Could you check a few things on this model? Use its own coordinates, in mm. Face numbers are marked on the shaded views. Round coordinates to 2 decimals unless told otherwise and drop trailing zeros. Loops run counter-clockwise (first coordinate to the right, second up) from the corner with the lowest first, then second, coordinate; pieces in that order, holes last. Notation, with made-up numbers: (51, 54) - (68, 54) arc R17 cw to (68, 82) - close; hole circle Ø9 at (83.5, -7.5). An arc over 180 degrees is marked (long way). Put each result on its own line as item: value. Start each with the question number.
from build123d import *

# Parameters (mm, degrees)
SKETCH1_R           = 46.5
SKETCH1_R_2         = 6.5
SKETCH1_R_3         = 10
SKETCH1_R_4         = 3.5
BOSS_EXTRUDE1_DEPTH = 2
SKETCH3_R           = 5
SKETCH3_R_2         = 3.5
BOSS_EXTRUDE2_DEPTH = 100
SKETCH4_R           = 30
SKETCH4_R_2         = 29
BOSS_EXTRUDE5_DEPTH = 2
FILLET2_R           = 2
SKETCH5_R           = 1
SKETCH5_R_2         = 3.5
CUT_EXTRUDE1_DEPTH  = 1
SKETCH6_R           = 2
CUT_EXTRUDE2_DEPTH  = 2
CHAMFER2_SIZE       = 0.8
SKETCH7_R           = 61.085714235
CUT_EXTRUDE3_DEPTH  = 122.361031637


with BuildPart() as part:
    # Sketch1 → Boss-Extrude1 (new body)
    with BuildSketch(Plane(origin=(0, 0, 0), x_dir=(1, 0, 0), z_dir=(0, 1, 0))):
        with Locations(Location((0, 0, 0), (0, 0, 270))):
            Circle(SKETCH1_R)
        with Locations(Location((0, 15, 0), (0, 0, 270))):
            Circle(SKETCH1_R_2, mode=Mode.SUBTRACT)
        with Locations(Location((-12.990381057, -7.5, 0), (0, 0, 270))):
            Circle(SKETCH1_R_3, mode=Mode.SUBTRACT)
        with Locations(Location((12.990381057, -7.5, 0), (0, 0, 270))):
            Circle(SKETCH1_R_4, mode=Mode.SUBTRACT)
        with Locations(Location((0, 0, 0), (0, 0, 270))):
            Circle(SKETCH1_R_4, mode=Mode.SUBTRACT)
    extrude(amount=BOSS_EXTRUDE1_DEPTH)

    # Sketch3 → Boss-Extrude2 (add)
    with BuildSketch(Plane(origin=(0, 2, 0), x_dir=(1, 0, 0), z_dir=(0, 1, 0))):
        with Locations(Location((0, 0, 0), (0, 0, 210))):
            Circle(SKETCH3_R)
        with Locations(Location((0, 0, 0), (0, 0, 270))):
            Circle(SKETCH3_R_2, mode=Mode.SUBTRACT)
    extrude(amount=BOSS_EXTRUDE2_DEPTH)

    # Sketch6 → Cut-Extrude2 (cut)
    with BuildSketch(Plane.XZ):
        with Locations(Location((0, 35, 0), (0, 0, 270))):
            Circle(SKETCH6_R)
        with Locations(Location((27.364101886, 21.822143065, 0), (0, 0, 270))):
            Circle(SKETCH6_R)
        with Locations(Location((34.122476926, -7.788232688, 0), (0, 0, 270))):
            Circle(SKETCH6_R)
        with Locations(Location((15.185930869, -31.533910377, 0), (0, 0, 270))):
            Circle(SKETCH6_R)
        with Locations(Location((-15.185930869, -31.533910377, 0), (0, 0, 270))):
            Circle(SKETCH6_R)
        with Locations(Location((-34.122476926, -7.788232688, 0), (0, 0, 270))):
            Circle(SKETCH6_R)
        with Locations(Location((-27.364101886, 21.822143065, 0), (0, 0, 270))):
            Circle(SKETCH6_R)
    extrude(amount=-CUT_EXTRUDE2_DEPTH, mode=Mode.SUBTRACT)

    # Chamfer2
    chamfer2_edges = [part.edges().sort_by_distance(p)[0] for p in [
        (12.990381057, 0, 4),
        (34.122476926, 0, -5.788232688),
        (27.364101886, 0, 23.822143065),
        (0, 0, 37),
        (-27.364101886, 0, 23.822143065),
        (-34.122476926, 0, -5.788232688),
        (-15.185930869, 0, -29.533910377),
        (15.185930869, 0, -29.533910377),
    ]]
    chamfer(chamfer2_edges, length=CHAMFER2_SIZE)

    # Sketch7 → Cut-Extrude3 (cut, through all)
    with BuildSketch(Plane.XZ.offset(-102)):
        Circle(SKETCH7_R)
    extrude(amount=CUT_EXTRUDE3_DEPTH, mode=Mode.SUBTRACT)


with BuildPart() as body_2:
    # Sketch4 → Boss-Extrude5 (new body)
    # profile 1 of 11: a face of its own
    with BuildSketch(Plane(origin=(0, 102, 0), x_dir=(1, 0, 0), z_dir=(0, 1, 0))):
        with Locations(Location((0, 0, 0), (0, 0, 270))):
            Circle(SKETCH4_R)
        Circle(SKETCH4_R_2, mode=Mode.SUBTRACT)
    # profile 2 of 11: a face of its own
    with BuildSketch(Plane(origin=(0, 102, 0), x_dir=(1, 0, 0), z_dir=(0, 1, 0))):
        with BuildLine():
            ThreePointArc((0.372035902, 9.373321886), (-3.288218135, 5.713067848), (-8.288218135, 4.373321886))
            Line((-8.288218135, 4.373321886), (-28.668345883, 4.373321886))
            ThreePointArc((-28.668345883, 4.373321886), (-29, 0), (-28.668345883, -4.373321886))
            Line((-28.668345883, -4.373321886), (-8.209333805, -4.373321886))
            ThreePointArc((-8.209333805, -4.373321886), (-3.209333805, -5.713067848), (0.450920232, -9.373321886))
            Line((0.450920232, -9.373321886), (10.619428606, -26.985695027))
            ThreePointArc((10.619428606, -26.985695027), (14.567551204, -25.075614687), (18.182472179, -22.591983212))
            Line((18.182472179, -22.591983212), (7.986293771, -4.931684166))
            ThreePointArc((7.986293771, -4.931684166), (6.646547809, 0.068315834), (7.986293771, 5.068315834))
            Line((7.986293771, 5.068315834), (18.128572143, 22.635257278))
            ThreePointArc((18.128572143, 22.635257278), (14.507755353, 25.110257558), (10.555107028, 27.010918452))
            Line((10.555107028, 27.010918452), (0.372035902, 9.373321886))
        make_face()
        with BuildLine():
            ThreePointArc((-4.421197961, -2.542244793), (-5.099992146, 0.008950407), (-4.412247554, 2.557747353))
            ThreePointArc((-4.412247554, 2.557747353), (-2.542244793, 4.421197961), (0.008950407, 5.099992146))
            ThreePointArc((0.008950407, 5.099992146), (2.557747353, 4.412247554), (4.421197961, 2.542244793))
            ThreePointArc((4.421197961, 2.542244793), (4.927378086, 1.315653905), (5.1, 0))
            ThreePointArc((5.1, 0), (4.925061549, -1.324299338), (4.412247554, -2.557747353))
            ThreePointArc((4.412247554, -2.557747353), (2.542244793, -4.421197961), (-0.008950407, -5.099992146))
            ThreePointArc((-0.008950407, -5.099992146), (-2.557747353, -4.412247554), (-4.421197961, -2.542244793))
        make_face(mode=Mode.SUBTRACT)
    # profile 3 of 11: a face of its own
    with BuildSketch(Plane(origin=(0, 102, 0), x_dir=(1, 0, 0), z_dir=(0, 1, 0))):
        with BuildLine():
            Line((-0.008950407, -5.099992146), (-0.008774909, -4.9999923))
            ThreePointArc((-0.008774909, -4.9999923), (-2.507595444, -4.325732896), (-4.334507805, -2.492396856))
            Line((-4.334507805, -2.492396856), (-4.421197961, -2.542244793))
            ThreePointArc((-4.421197961, -2.542244793), (-2.557747353, -4.412247554), (-0.008950407, -5.099992146))
        make_face()
    # profile 4 of 11: a face of its own
    with BuildSketch(Plane(origin=(0, 102, 0), x_dir=(1, 0, 0), z_dir=(0, 1, 0))):
        with BuildLine():
            Line((-4.412247554, 2.557747353), (-4.325732896, 2.507595444))
            ThreePointArc((-4.325732896, 2.507595444), (-2.492396856, 4.334507805), (0.008774909, 4.9999923))
            Line((0.008774909, 4.9999923), (0.008950407, 5.099992146))
            ThreePointArc((0.008950407, 5.099992146), (-2.542244793, 4.421197961), (-4.412247554, 2.557747353))
        make_face()
    # profile 5 of 11: a face of its own
    with BuildSketch(Plane(origin=(0, 102, 0), x_dir=(1, 0, 0), z_dir=(0, 1, 0))):
        with BuildLine():
            Line((4.421197961, 2.542244793), (4.334507805, 2.492396856))
            ThreePointArc((4.334507805, 2.492396856), (4.830762829, 1.28985677), (5, 0))
            ThreePointArc((5, 0), (4.828491715, -1.298332685), (4.325732896, -2.507595444))
            Line((4.325732896, -2.507595444), (4.412247554, -2.557747353))
            ThreePointArc((4.412247554, -2.557747353), (4.925061549, -1.324299338), (5.1, 0))
            ThreePointArc((5.1, 0), (4.927378086, 1.315653905), (4.421197961, 2.542244793))
        make_face()
    # profile 6 of 11: a face of its own
    with BuildSketch(Plane(origin=(0, 102, 0), x_dir=(1, 0, 0), z_dir=(0, 1, 0))):
        with BuildLine():
            ThreePointArc((-4.334507805, -2.492396856), (-4.9999923, 0.008774909), (-4.325732896, 2.507595444))
            Line((-4.325732896, 2.507595444), (-4.412247554, 2.557747353))
            ThreePointArc((-4.412247554, 2.557747353), (-5.099992146, 0.008950407), (-4.421197961, -2.542244793))
            Line((-4.421197961, -2.542244793), (-4.334507805, -2.492396856))
        make_face()
    # profile 7 of 11: a face of its own
    with BuildSketch(Plane(origin=(0, 102, 0), x_dir=(1, 0, 0), z_dir=(0, 1, 0))):
        with BuildLine():
            Line((4.412247554, -2.557747353), (4.325732896, -2.507595444))
            ThreePointArc((4.325732896, -2.507595444), (2.492396856, -4.334507805), (-0.008774909, -4.9999923))
            Line((-0.008774909, -4.9999923), (-0.008950407, -5.099992146))
            ThreePointArc((-0.008950407, -5.099992146), (2.542244793, -4.421197961), (4.412247554, -2.557747353))
        make_face()
    # profile 8 of 11: a face of its own
    with BuildSketch(Plane(origin=(0, 102, 0), x_dir=(1, 0, 0), z_dir=(0, 1, 0))):
        with BuildLine():
            Line((0.008950407, 5.099992146), (0.008774909, 4.9999923))
            ThreePointArc((0.008774909, 4.9999923), (2.507595444, 4.325732896), (4.334507805, 2.492396856))
            Line((4.334507805, 2.492396856), (4.421197961, 2.542244793))
            ThreePointArc((4.421197961, 2.542244793), (2.557747353, 4.412247554), (0.008950407, 5.099992146))
        make_face()
    # profile 9 of 11: a face of its own
    with BuildSketch(Plane(origin=(0, 102, 0), x_dir=(1, 0, 0), z_dir=(0, 1, 0))):
        with BuildLine():
            Line((-4.325732896, 2.507595444), (-3.028013027, 1.755316811))
            ThreePointArc((-3.028013027, 1.755316811), (-1.744677799, 3.034155464), (0.006142436, 3.49999461))
            Line((0.006142436, 3.49999461), (0.008774909, 4.9999923))
            ThreePointArc((0.008774909, 4.9999923), (-2.492396856, 4.334507805), (-4.325732896, 2.507595444))
        make_face()
    # profile 10 of 11: a face of its own
    with BuildSketch(Plane(origin=(0, 102, 0), x_dir=(1, 0, 0), z_dir=(0, 1, 0))):
        with BuildLine():
            Line((-0.008774909, -4.9999923), (-0.006142436, -3.49999461))
            ThreePointArc((-0.006142436, -3.49999461), (-1.755316811, -3.028013027), (-3.034155464, -1.744677799))
            Line((-3.034155464, -1.744677799), (-4.334507805, -2.492396856))
            ThreePointArc((-4.334507805, -2.492396856), (-2.507595444, -4.325732896), (-0.008774909, -4.9999923))
        make_face()
    # profile 11 of 11: a face of its own
    with BuildSketch(Plane(origin=(0, 102, 0), x_dir=(1, 0, 0), z_dir=(0, 1, 0))):
        with BuildLine():
            Line((4.334507805, 2.492396856), (3.034155464, 1.744677799))
            ThreePointArc((3.034155464, 1.744677799), (3.38153398, 0.902899739), (3.5, 0))
            ThreePointArc((3.5, 0), (3.3799442, -0.908832879), (3.028013027, -1.755316811))
            Line((3.028013027, -1.755316811), (4.325732896, -2.507595444))
            ThreePointArc((4.325732896, -2.507595444), (4.828491715, -1.298332685), (5, 0))
            ThreePointArc((5, 0), (4.830762829, 1.28985677), (4.334507805, 2.492396856))
        make_face()
    extrude(amount=BOSS_EXTRUDE5_DEPTH)

    # Fillet2
    fillet2_edges = [body_2.edges().sort_by_distance(p)[0] for p in [
        (10.555107028, 103, -27.010918452),
        (-28.668345883, 103, -4.373321886),
        (18.128572143, 103, -22.635257278),
        (18.182472179, 103, 22.591983212),
        (10.619428606, 103, 26.985695027),
        (-28.668345883, 103, 4.373321886),
    ]]
    fillet(fillet2_edges, radius=FILLET2_R)

    # Sketch5 → Cut-Extrude1 (cut)
    with BuildSketch(Plane.XZ.offset(-102)):
        with Locations(Location((-15, 0, 0), (0, 0, 270))):
            Circle(SKETCH5_R)
        with Locations(Location((7.5, 12.990381057, 0), (0, 0, 270))):
            Circle(SKETCH5_R_2)
        Polygon((8.383974596, -16.52146997), (4.883974596, -10.459292144), (6.616025404, -9.459292144), (10.116025404, -15.52146997), align=None)
    extrude(amount=-CUT_EXTRUDE1_DEPTH, mode=Mode.SUBTRACT)


solid = body_2.part
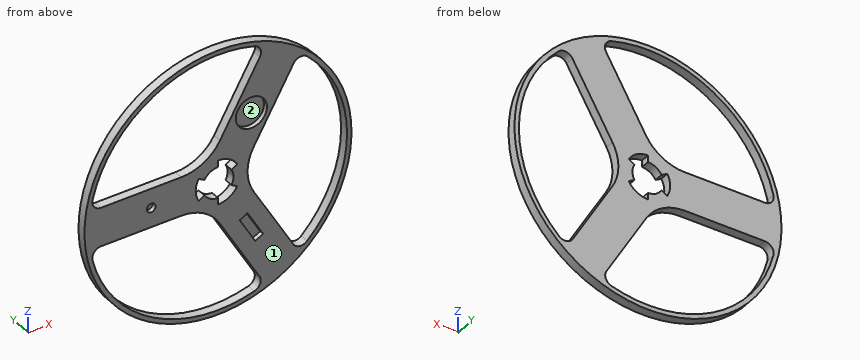
Item 1: Suppose I cut it at B-B, the plane z = 6. List the corners of the cut face in (x, y) for me.
Item 2: Suppose I cut it at C-C, the plane x = -15. List the corners of the cut face in (y, z) for me.
Item 3: Suppose I cut it at A-A, the plane x = -6. List the corners of the cut face in (y, z) for me, then the cut area to 3 significant figures.
Item 4: Thinking about a two-plate mould opening in X: for the marked faces 1 and 2, which applies, released by +X, released by -X, zero draft, split by the parting line, or undercut?
Item 5: Will these pins go through, and if not, where does the flat tip stop? P1, Ø5.5, axis at x = 7, z = 12.5, coming from the -Y side; P2, Ø2.5, axis at x = 7, z = -12.5, coming from the -Y side; P3, Ø1, axis at y = 103, z = 6.5, coming from the -X side.
Item 6: I need wall thicknesses on line 1 (X direction, y = 102.5, z = 17); line 2 (Z direction, x = 8.5, y = 103.5); line 3 (Z direction, x = -18, y = 102.1). Which ranges of each line are inside material? Lowest first, please. Write a range as from..to.
Numbers:
1. outline: (-29.39, 102) - (-28.2, 102) - (-28.2, 104) - (-29.39, 104) - close; (-2.74, 102) - (8.6, 102) - (8.6, 104) - (-2.74, 104) - close; (28.37, 102) - (29.39, 102) - (29.39, 104) - (28.37, 104) - close
2. outline: (102, -25.98) - (104, -25.98) - (104, -24.82) - (102, -24.82) - close; (102, -4.37) - (104, -4.37) - (104, 4.37) - (102, 4.37) - (102, 1) - (103, 1) - (103, -1) - (102, -1) - close; (102, 24.82) - (104, 24.82) - (104, 25.98) - (102, 25.98) - close
3. outline: (102, -29.39) - (104, -29.39) - (104, -28.37) - (102, -28.37) - close; (102, -4.64) - (104, -4.64) - (104, 4.62) - (102, 4.62) - close; (102, 28.37) - (104, 28.37) - (104, 29.39) - (102, 29.39) - close
3. area: 22.6 mm^2
4. face 1: zero draft
4. face 2: undercut
5. P1: y = 103
5. P2: y = 102
5. P3: x = -29.39
6. line 1: -24.72..-23.49, 4.85..14.95, 23.49..24.72
6. line 2: -28.77..-27.7, -23.45..-5.96, 5.82..23.31, 27.71..28.77
6. line 3: -24..-22.74, -4.37..4.37, 22.74..24
